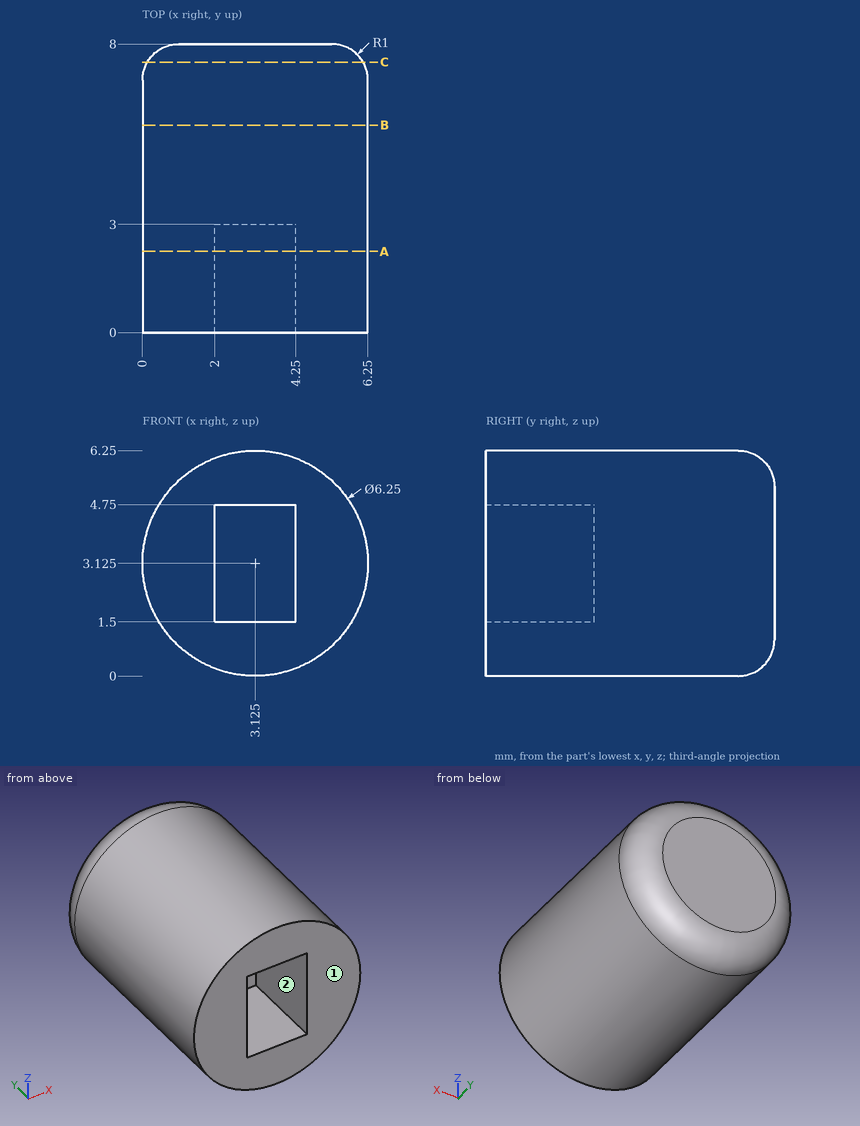
Study the drawing (mm; zero at the part's minimum x, y, z) and answer. A direction names the side the tool comes from. Give positions to 0.01 mm unless a question says otherwise; leave off trailing zeros. Order: outer loops, then holes, each group sorted by start corner. A loop starts at its lowest first (then second) coordinate and runs counter-clockwise, first axis right, second up. Notation, with made-up numbers: (62.5, -26) -> (74.5, -26) arc R21 ccw to (74.5, -6) -> close; hole circle Ø5 at (27.25, 27). An arc over 180 degrees is marked (long way). Put each result on its own line as item: value.
Item 1: A cutting plane is placed at C-C on y = 7.5. Give the vertices of the cut face in (x, z) (3 decimals).
Established:
outline: circle Ø5.982 at (3.125, 3.125)
Item 2: Given P1, Ø2, axis at x = 5, y = 2, coming from the +Z side (3 decimals); P2, Ø1, axis at y = 5.5, z = 4, coming from the -X side; P3, Ø3, axis at x = 3, y = 6.5, coming from the +Z side; P4, Ø0.7, axis at x = 3, z = 3, coming from the -Y side, each flat-ended and moving along its own axis, determine where each tip first touches the part or whether it passes through.
Established:
P1: stops at z = 6.125
P2: stops at x = 0.02
P3: stops at z = 6.25
P4: stops at y = 3
Item 3: A cutting plane is placed at A-A on y = 2.25. Give the vertices of the cut face in (x, z) (3 decimals), plus the area to 3 significant figures.
Established:
outline: circle Ø6.25 at (3.125, 3.125); hole (2, 1.5) -> (4.25, 1.5) -> (4.25, 4.75) -> (2, 4.75) -> close
area: 23.4 mm^2
Item 4: For the marked faces 1 and 2, determine the directions among +Z, -Z, +X, -X, +Y, -Y from which every point of the face is accessible in a straight line to the end or side of a thin tool.
Established:
face 1: +Z, -Z, +X, -X, -Y
face 2: -Y
Item 5: Straight lines are drawn through the part: line 1 (Y direction, x = 3, z = 4.5); line 2 (Z direction, x = 3.25, y = 3.75); line 3 (Z direction, x = 3, y = 1.25). For each, find the intervals that lie inside material, in ascending order.
Established:
line 1: y = 3 to 8
line 2: z = 0 to 6.25
line 3: z = 0 to 1.5, 4.75 to 6.25
Item 6: A cutting plane is placed at B-B on y = 5.75. Give the vertices of the cut face in (x, z) (3 decimals).
Established:
outline: circle Ø6.25 at (3.125, 3.125)
